Input: part model. Units: mm. Frame: model coordinates. A direction names the side the tool comes from. Coordinates: 2 decimals unless noted, no trailing zeros. Order: outer loops, then holes, each group sorted by start corner. A loop starts at its lowest first (then second) coordinate and runs counter-clockwise, first axis right, second up. Notation, with made-up numbers: (56.5, -6.75) - (108.5, -6.75) arc R24 cw to (108.5, 27.25) - close; hole circle Ø5 at (89.5, -25.75). An arc over 180 degrees is marked (long way). Use a Markdown table: item, result. Add a question column.
from build123d import *

# Parameters (mm, degrees)
ESQUISSE1_W                  = 120
ESQUISSE1_H                  = 200
BOSS_EXTRU_2_DEPTH           = 25
ESQUISSE3_W                  = 120
ESQUISSE3_H                  = 40
BOSS_EXTRU_3_DEPTH           = 70
CONG_1_R                     = 15
ESQUISSE4_W                  = 120
ESQUISSE4_H                  = 40
BOSS_EXTRU_4_DEPTH           = 140
CONG_2_R                     = 30
ESQUISSE5_W                  = 50
ESQUISSE5_H                  = 30
BOSS_EXTRU_9_DEPTH           = 7.5
ESQUISSE7_W                  = 100
ESQUISSE7_H                  = 80
ENL_V_MAT_EXTRU_1_DEPTH      = 35
ENL_V_MAT_EXTRU_7_REACH      = 262
ESQUISSE8_R                  = 7.5
ESQUISSE12_W                 = 50
ESQUISSE12_H                 = 30
ENL_V_MAT_EXTRU_8_DEPTH      = 5
ESQUISSE13_R                 = 12.5
ENL_V_MAT_EXTRU_9_DEPTH      = 1
ENL_V_MAT_EXTRU_9_DEPTH_BACK = 121
ESQUISSE14_W                 = 15
ESQUISSE14_H                 = 5
ENL_V_MAT_EXTRU_10_DEPTH     = 3
ESQUISSE22_W                 = 142.933359841
ESQUISSE22_H                 = 230.615168818
ENL_V_MAT_EXTRU_12_DEPTH     = 141
ESQUISSE23_W                 = 105
ESQUISSE23_H                 = 150
ENL_V_MAT_EXTRU_13_DEPTH     = 12.5
ESQUISSE24_R                 = 1.25
ENL_V_MAT_EXTRU_14_DEPTH     = 5
CONG_4_R                     = 15
ESQUISSE25_W                 = 11
ESQUISSE25_H                 = 200
ENL_V_MAT_EXTRU_15_DEPTH     = 121
ESQUISSE26_R                 = 5
ENL_V_MAT_EXTRU_16_DEPTH     = 11
ESQUISSE28_W                 = 34
ESQUISSE28_H                 = 40
ENL_V_MAT_EXTRU_17_DEPTH     = 121
CONG_5_R                     = 20
ESQUISSE29_R                 = 1.25
ENL_V_MAT_EXTRU_18_DEPTH     = 4
ESQUISSE30_R                 = 1.25
ENL_V_MAT_EXTRU_19_DEPTH     = 121


with BuildPart() as part:
    # Esquisse1 → Boss.-Extru.2 (new body, symmetric)
    with BuildSketch(Plane.XY):
        with Locations((60, 100)):
            Rectangle(ESQUISSE1_W, ESQUISSE1_H)
    extrude(amount=BOSS_EXTRU_2_DEPTH, both=True)

    # Esquisse3 → Boss.-Extru.3 (add)
    with BuildSketch(Plane.XY.offset(25)):
        with Locations((60, 20)):
            Rectangle(ESQUISSE3_W, ESQUISSE3_H)
    extrude(amount=BOSS_EXTRU_3_DEPTH)

    # Congé1
    cong_1_edges = [part.edges().sort_by_distance(p)[0] for p in [
        (60, 40, 25),
    ]]
    fillet(cong_1_edges, radius=CONG_1_R)

    # Esquisse4 → Boss.-Extru.4 (add)
    with BuildSketch(Plane(origin=(0, 0, -25), x_dir=(-1, 0, 0), z_dir=(0, 0, -1))):
        with Locations((-60, 20)):
            Rectangle(ESQUISSE4_W, ESQUISSE4_H)
    extrude(amount=BOSS_EXTRU_4_DEPTH)

    # Congé2
    cong_2_edges = [part.edges().sort_by_distance(p)[0] for p in [
        (60, 40, -25),
    ]]
    fillet(cong_2_edges, radius=CONG_2_R)

    # Esquisse5 → Boss.-Extru.9 (add)
    with BuildSketch(Plane.XY.offset(95)):
        with Locations((60, 20)):
            Rectangle(ESQUISSE5_W, ESQUISSE5_H)
    extrude(amount=-BOSS_EXTRU_9_DEPTH)

    # Esquisse7 → Enlèv. mat.-Extru.1 (cut)
    with BuildSketch(Plane.XZ):
        with Locations((60, 45)):
            Rectangle(ESQUISSE7_W, ESQUISSE7_H)
    extrude(amount=-ENL_V_MAT_EXTRU_1_DEPTH, mode=Mode.SUBTRACT)

    # Esquisse8 → Enlèv. mat.-Extru.7 (cut, up to next)
    with BuildSketch(Plane.XY.offset(95), mode=Mode.PRIVATE) as enl_v_mat_extru_7_sk1:
        with Locations((47.5, 20)):
            Circle(ESQUISSE8_R)
    enl_v_mat_extru_7_tool1 = extrude(enl_v_mat_extru_7_sk1.sketch, amount=-ENL_V_MAT_EXTRU_7_REACH, mode=Mode.PRIVATE) & part.part
    add(enl_v_mat_extru_7_tool1.solids().sort_by_distance((47.5, 20, 95))[0], mode=Mode.SUBTRACT)
    # Esquisse8 → Enlèv. mat.-Extru.7 (cut, up to next)
    with BuildSketch(Plane.XY.offset(95), mode=Mode.PRIVATE) as enl_v_mat_extru_7_sk2:
        with Locations((72.5, 20)):
            Circle(ESQUISSE8_R)
    enl_v_mat_extru_7_tool2 = extrude(enl_v_mat_extru_7_sk2.sketch, amount=-ENL_V_MAT_EXTRU_7_REACH, mode=Mode.PRIVATE) & part.part
    add(enl_v_mat_extru_7_tool2.solids().sort_by_distance((72.5, 20, 95))[0], mode=Mode.SUBTRACT)

    # Esquisse12 → Enlèv. mat.-Extru.8 (cut)
    with BuildSketch(Plane(origin=(0, 0, 85), x_dir=(-1, 0, 0), z_dir=(0, 0, -1))):
        with Locations((-60, 20)):
            Rectangle(ESQUISSE12_W, ESQUISSE12_H)
    extrude(amount=-ENL_V_MAT_EXTRU_8_DEPTH, mode=Mode.SUBTRACT)

    # Esquisse13 → Enlèv. mat.-Extru.9 (cut, two sides)
    with BuildSketch(Plane(origin=(120, 0, 0), x_dir=(0, 0, -1), z_dir=(1, 0, 0))) as enl_v_mat_extru_9_sk:
        with Locations((-60, 20)):
            Circle(ESQUISSE13_R)
    extrude(amount=ENL_V_MAT_EXTRU_9_DEPTH, mode=Mode.SUBTRACT)
    extrude(enl_v_mat_extru_9_sk.sketch, amount=-ENL_V_MAT_EXTRU_9_DEPTH_BACK, mode=Mode.SUBTRACT)

    # Esquisse14 → Enlèv. mat.-Extru.10 (cut)
    with BuildSketch(Plane(origin=(0, 0, 85), x_dir=(-1, 0, 0), z_dir=(0, 0, -1))):
        with Locations((-60, 2.5)):
            Rectangle(ESQUISSE14_W, ESQUISSE14_H)
    extrude(amount=-ENL_V_MAT_EXTRU_10_DEPTH, mode=Mode.SUBTRACT)

    # Esquisse22 → Enlèv. mat.-Extru.12 (cut)
    with BuildSketch(Plane.XY):
        with Locations((64.967602161, 91.924485341)):
            Rectangle(ESQUISSE22_W, ESQUISSE22_H)
    extrude(amount=ENL_V_MAT_EXTRU_12_DEPTH, mode=Mode.SUBTRACT)

    # Esquisse23 → Enlèv. mat.-Extru.13 (cut)
    with BuildSketch(Plane.XY):
        with Locations((60, 117.5)):
            Rectangle(ESQUISSE23_W, ESQUISSE23_H)
    extrude(amount=-ENL_V_MAT_EXTRU_13_DEPTH, mode=Mode.SUBTRACT)

    # Esquisse24 → Enlèv. mat.-Extru.14 (cut)
    with BuildSketch(Plane(origin=(0, 0, 0), x_dir=(-1, 0, 0), z_dir=(0, -1, 0))):
        with Locations((-76.322658076, 105)):
            Circle(ESQUISSE24_R)
        with Locations((-46.322658076, 105)):
            Circle(ESQUISSE24_R)
        with Locations((-45, 85)):
            Circle(ESQUISSE24_R)
        with Locations((-75, 85)):
            Circle(ESQUISSE24_R)
    extrude(amount=-ENL_V_MAT_EXTRU_14_DEPTH, mode=Mode.SUBTRACT)

    # Congé4
    cong_4_edges = [part.edges().sort_by_distance(p)[0] for p in [
        (120, 200, -12.5),
        (0, 200, -12.5),
        (60, 40, -165),
    ]]
    fillet(cong_4_edges, radius=CONG_4_R)

    # Esquisse25 → Enlèv. mat.-Extru.15 (cut, through all)
    with BuildSketch(Plane(origin=(0, 0, 0), x_dir=(0, 0, -1), z_dir=(1, 0, 0))):
        with Locations((5.5, 100)):
            Rectangle(ESQUISSE25_W, ESQUISSE25_H)
    extrude(amount=ENL_V_MAT_EXTRU_15_DEPTH, mode=Mode.SUBTRACT)

    # Esquisse26 → Enlèv. mat.-Extru.16 (cut)
    with BuildSketch(Plane.XY.offset(-12.5)):
        with Locations((15.5, 145.5)):
            Circle(ESQUISSE26_R)
        with Locations((15.5, 133.5)):
            Circle(ESQUISSE26_R)
    extrude(amount=-ENL_V_MAT_EXTRU_16_DEPTH, mode=Mode.SUBTRACT)

    # Esquisse28 → Enlèv. mat.-Extru.17 (cut, through all)
    with BuildSketch(Plane(origin=(120, 0, 0), x_dir=(0, 0, -1), z_dir=(1, 0, 0))):
        with Locations((148, 20)):
            Rectangle(ESQUISSE28_W, ESQUISSE28_H)
    extrude(amount=-ENL_V_MAT_EXTRU_17_DEPTH, mode=Mode.SUBTRACT)

    # Congé5
    cong_5_edges = [part.edges().sort_by_distance(p)[0] for p in [
        (60, 40, -131),
    ]]
    fillet(cong_5_edges, radius=CONG_5_R)

    # Esquisse29 → Enlèv. mat.-Extru.18 (cut)
    with BuildSketch(Plane.XY.offset(-11)):
        with Locations((60, 20)):
            Circle(ESQUISSE29_R)
    extrude(amount=-ENL_V_MAT_EXTRU_18_DEPTH, mode=Mode.SUBTRACT)

    # Esquisse30 → Enlèv. mat.-Extru.19 (cut, through all)
    with BuildSketch(Plane.XY.offset(-11)):
        with Locations((3.5, 110)):
            Circle(ESQUISSE30_R)
        with Locations((116.5, 110)):
            Circle(ESQUISSE30_R)
        with Locations((60, 195.964841854)):
            Circle(ESQUISSE30_R)
    extrude(amount=-ENL_V_MAT_EXTRU_19_DEPTH, mode=Mode.SUBTRACT)


solid = part.part
1) Contact query for flat-ended pins moving along their axis: P1, Ø13, axis at x = 15.5, y = 145.5, coming from the -Z side; P2, Ø0.8, axis at x = 45.5, z = -85.5, coming from the -Y side; P3, Ø8, axis at x = 96.5, y = 77, coming from the +Z side; P4, Ø8, axis at y = 97, z = -27, coming from the +X side. Output: stop coordinate, or through.
2) Cut plane D-D (z = -50.5). Return the cut outline in (x, y).
3) Pull-direction query (Y, two-part tool) for faces 4 (the flat face through (120, 37, -57)), 5 (the cylindrical face through (59.16, 33.986, -125.297)), 6 (the cylindrical face through (17.807, 141.064, -17.923)); classes: pulls with the +Y half, pulls with the -Y half, needs draft (parallel to the pull), parting line crosses it, or undercut.
4) Material intervals for L1, parallel to X at y = 110, z = -16; L2, parallel to X at y = 1, z = -105; L3, parallel to Y at x = 60, z = -20.5, sorted ascending.
5) Cut plane C-C (y = 95). Return the cut outline in (x, z).
6) Cut plane A-A (y = 145.5). Return the cut outline in (x, z).
7) Cut plane B-B (z = -66.5). Return the cut outline in (x, y), and give its area (3 significant figures).
8) Reachability of faces 1 (the flat face through (15, 134, -23.5)), 2 (the flat face through (59, 136, -25)), 3 (the cylindrical face through (4.51, 195.72, -18.1)) from +Z, -Z, +X, -X, +Y, -Y: full face, straight path, thin tool, end or side. Return the list, or none.
Computed:
| question | item | result |
|---|---|---|
| 1 | P1 | stops at z = -25 |
| 1 | P2 | stops at y = 5 |
| 1 | P3 | stops at z = -12.5 |
| 1 | P4 | stops at x = 120 |
| 2 | outline | (0, 0) - (120, 0) - (120, 40.34) - (0, 40.34) - close |
| 3 | face 4 | needs draft |
| 3 | face 5 | pulls with the +Y half |
| 3 | face 6 | undercut |
| 4 | L1 | x = 0 to 2.25, 4.75 to 115.25, 117.75 to 120 |
| 4 | L2 | x = 0 to 45.07, 47.57 to 75.07, 77.57 to 120 |
| 4 | L3 | y = 0 to 194.71, 197.21 to 200 |
| 5 | outline | (0, -25) - (120, -25) - (120, -11) - (112.5, -11) - (112.5, -12.5) - (7.5, -12.5) - (7.5, -11) - (0, -11) - close |
| 6 | outline | (0, -25) - (120, -25) - (120, -11) - (112.5, -11) - (112.5, -12.5) - (20.5, -12.5) - (20.5, -23.5) - (10.5, -23.5) - (10.5, -12.5) - (7.5, -12.5) - (7.5, -11) - (0, -11) - close |
| 7 | outline | (0, 0) - (120, 0) - (120, 40) - (0, 40) - close |
| 7 | area | 4,800 mm2 |
| 8 | face 1 | +Z |
| 8 | face 2 | -Z, +X, -X, +Y |
| 8 | face 3 | +Z, -Z, -X, +Y |
